from build123d import *

# Parameters (mm, degrees)
F0_R     = 1.6
F1_DEPTH = 2
F3_W     = 18
F3_H     = 35.5
F4_DEPTH = 17
F6_W     = 8
F6_H     = 3
F7_DEPTH = 2


with BuildPart() as f1:
    # F0 (on Top) → F1 (new body)
    with BuildSketch(Plane.XY):
        with BuildLine():
            Line((-40.07, -33.78), (40.07, -33.78))
            Line((40.07, -33.78), (40.07, 33.78))
            Line((40.07, 33.78), (0.5, 33.78))
            ThreePointArc((0.5, 33.78), (0, 33.28), (-0.5, 33.78))
            Line((-0.5, 33.78), (-40.07, 33.78))
            Line((-40.07, 33.78), (-40.07, -33.78))
        make_face()
        with Locations((-37.53, -31.24)):
            Circle(F0_R, mode=Mode.SUBTRACT)
        with Locations((37.53, -31.24)):
            Circle(F0_R, mode=Mode.SUBTRACT)
        with Locations((-37.53, 31.24)):
            Circle(F0_R, mode=Mode.SUBTRACT)
        with Locations((37.53, 31.24)):
            Circle(F0_R, mode=Mode.SUBTRACT)
        with BuildLine():
            ThreePointArc((-0.5, 33.78), (0, 33.28), (0.5, 33.78))
            Line((0.5, 33.78), (-0.5, 33.78))
        make_face()
        with BuildLine():
            Line((-0.5, 33.78), (0.5, 33.78))
            ThreePointArc((0.5, 33.78), (0, 34.28), (-0.5, 33.78))
        make_face()
    extrude(amount=F1_DEPTH)

    # F3 (on offset) → F4 (join)
    with BuildSketch(Plane.XY.offset(2)):
        with Locations((14.56, 16.03)):
            Rectangle(F3_W, F3_H)
    extrude(amount=F4_DEPTH)

    # F6 (on offset) → F7 (join)
    with BuildSketch(Plane(origin=(0, 33.78, 0), x_dir=(-1, 0, 0), z_dir=(0, 1, 0))):
        with Locations((-14.56, 17.5)):
            Rectangle(F6_W, F6_H)
    extrude(amount=F7_DEPTH)


solid = f1.part
CAD build for the part. Positions are in the model's coordinates, mm. A direction names the side the tool comes from. Give positions to 0.01 mm unless a question says otherwise; leave off trailing zeros. Write each loop counter-clockwise with the first axis right and the second up, starting at its lowest first coordinate (ties: lowest second). Pieces come first, ordered by that corner, then holes. Notation, with made-up numbers: (0, 34) -> (15, 34) arc R18 ccw to (15, 60) -> close; hole circle Ø6 at (0.25, 36). An arc over 180 degrees is marked (long way). Return JSON: item names as keys, results as strings.
Item 1: Band-saw the part on C-C (y = -31.24). List the corners of the cut face in (x, z).
Answer below:
{"outline": "(-40.07, 0) -> (-39.13, 0) -> (-39.13, 2) -> (-40.07, 2) -> close; (-35.93, 0) -> (35.93, 0) -> (35.93, 2) -> (-35.93, 2) -> close; (39.13, 0) -> (40.07, 0) -> (40.07, 2) -> (39.13, 2) -> close"}
Item 2: Tool access for faces 4 (the flat face through (14, -1.72, 10)), 5 (the flat face through (23.56, 16, 10)), 6 (the flat face through (18.56, 35, 17)): list every direction of +Z, -Z, +X, -X, +Y, -Y with a clear straight run to the whole face (end or side of a thin tool).
Answer below:
{"face 4": "+Z, +X, -X, -Y", "face 5": "+Z, +X, +Y, -Y", "face 6": "+Z, -Z, +X, +Y"}
Item 3: Band-saw the part on A-A (z = 17). List the corners of the cut face in (x, y).
Answer below:
{"outline": "(5.56, -1.72) -> (23.56, -1.72) -> (23.56, 33.78) -> (18.56, 33.78) -> (18.56, 35.78) -> (10.56, 35.78) -> (10.56, 33.78) -> (5.56, 33.78) -> close"}
Item 4: Drop flat-ended pins along their axis: pin 1 (2 mm diameter, centred on x = 14, y = -15, fed in from +Z); pin 2 (2 mm diameter, centred on x = 15.5, y = 35, fed in from -Z); pin 3 (2 mm diameter, centred on y = 34.5, z = 18, fed in from +X). Give the stop position or say it passes through.
Answer below:
{"pin 1": "stops at z = 2", "pin 2": "stops at z = 16", "pin 3": "stops at x = 23.56"}
Item 5: Two-plate mould, pull along X, no slides. Class faces 1 (the flat face through (-40.07, 0, 1)), 2 (the flat face through (16, 33.78, 7)), 3 (the cylindrical face through (-37.88, -32.8, 0.99)): +X half, -X half, draft (parallel to the pull), parting line (faces both ways), or undercut.
Answer below:
{"face 1": "-X half", "face 2": "draft", "face 3": "undercut"}
Item 6: Band-saw the part on D-D (y = 6.5). List the corners of the cut face in (x, z).
Answer below:
{"outline": "(-40.07, 0) -> (40.07, 0) -> (40.07, 2) -> (23.56, 2) -> (23.56, 19) -> (5.56, 19) -> (5.56, 2) -> (-40.07, 2) -> close"}
Item 7: Drill centre lines: probe 1 along Y at (x, z) = (37.53, 1.1); probe 2 along Z at (x, y) = (17, -4); probe 3 along Y at (x, z) = (-3.5, 1.25). Where is each one in solid material? Low to high.
Answer below:
{"probe 1": "y = -33.78 to -32.84, -29.64 to 29.64, 32.84 to 33.78", "probe 2": "z = 0 to 2", "probe 3": "y = -33.78 to 33.78"}
Item 8: Band-saw the part on B-B (x = 37.53). List the corners of the cut face in (y, z).
Answer below:
{"outline": "(-33.78, 0) -> (-32.84, 0) -> (-32.84, 2) -> (-33.78, 2) -> close; (-29.64, 0) -> (29.64, 0) -> (29.64, 2) -> (-29.64, 2) -> close; (32.84, 0) -> (33.78, 0) -> (33.78, 2) -> (32.84, 2) -> close"}
